For this review, take the finished solid that the model builds, in its own axes (mm). Face numbers are marked on the shaded views. A direction names the side the tool comes from. Coordinates: 2 decimals unless noted, no trailing zeros. Loops run counter-clockwise (first coordinate to the right, second up) from the corner with the lowest first, then second, coordinate; pieces in that order, holes last. Notation, with made-up numbers: M -30,49.5 L 7,49.5 A29 cw 7,70.5 Z; hole C 57,78.25 d7. An arc over 180 degrees is marked long. Answer as a JSON object with one key per item and string values. Group by question number.
Item 1: Mouldability with a two-part tool opening along X and no side actions: class the marked faces 3, 4 and 5 as +X half, -X half, draft (parallel to the pull), parting line (faces both ways), or undercut.
Item 2: Add section B-B (y = -4). State the section outline as (x, z) points, then the cut area to 3 significant figures.
Item 3: Wall thickness on L1, parallel to X at y = -6, z = 22.25; L2, parallel to Y at x = -2, z = 5; L3, parallel to X at y = -2.5, z = 27.25: over which ranges is each line inside the solid? List them lowest first. Write a range as from..to.
Item 4: Add section A-A (z = 10.5). State the section outline as (x, y) points.
Item 5: Add section D-D (z = 6.75). State the section outline as (x, y) points.
Item 6: Add section C-C (y = 0). State the section outline as (x, z) points, then the cut area to 3 significant figures.
Item 7: Tool access review of the marked faces 1 and 2: name each direction out of +Z, -Z, +X, -X, +Y, -Y from which nothing blocks a thin tool from reaching the whole face with its end or side.
Item 8: Insertion check: pin 1 (15 mm diameter, centred on x = -4, z = 17, fed in from -Y); pin 2 (9 mm diameter, centred on x = -13, z = 10.5, fed in from +Y); pin 3 (3.5 mm diameter, centred on x = -22, y = 0.5, fed in from +Z). Each pin has a flat end and moves straight along its axis. Give the tip position at first contact, or say it passes through.
from build123d import *

# Parameters (mm, degrees)
BOSS_EXTRUDE1_DEPTH = 30
SKETCH3_W           = 6
SKETCH3_H           = 3
BOSS_EXTRUDE2_DEPTH = 10
SKETCH4_R           = 3.5
BOSS_EXTRUDE3_DEPTH = 30


with BuildPart() as part:
    # Sketch2 → Boss-Extrude1 (new body)
    with BuildSketch(Plane.XY):
        Polygon((-20, -1.5), (8.5, -1.5), (8.5, -8.5), (10.5, -8.5), (10.5, -1.5), (18, -1.5), (18, -8.5), (20, -8.5), (20, -1.5), (20, 1.5), (-20, 1.5), align=None)
    extrude(amount=BOSS_EXTRUDE1_DEPTH)

    # Sketch3 → Boss-Extrude2 (add)
    with BuildSketch(Plane.XY):
        with Locations((-23, 0)):
            Rectangle(SKETCH3_W, SKETCH3_H)
    extrude(amount=BOSS_EXTRUDE2_DEPTH)

    # Sketch4 → Boss-Extrude3 (add)
    with BuildSketch(Plane.XY):
        with Locations((-27.465142918, 0)):
            Circle(SKETCH4_R)
    extrude(amount=BOSS_EXTRUDE3_DEPTH)


solid = part.part
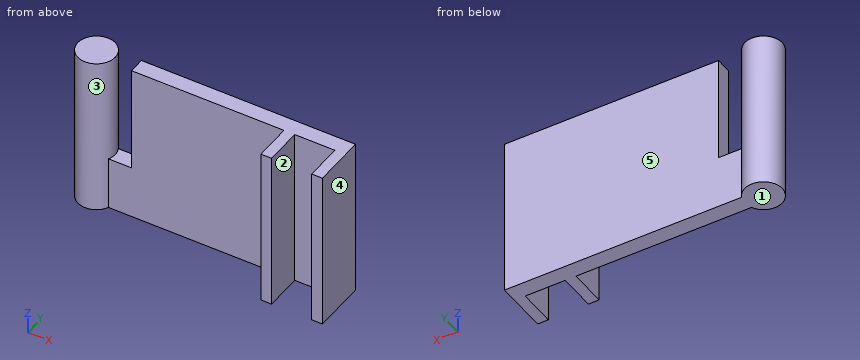
From the geometry:
{
 "1": {"face 3": "undercut", "face 4": "+X half", "face 5": "draft"},
 "2": {"outline": "M 8.5,0 L 10.5,0 L 10.5,30 L 8.5,30 Z; M 18,0 L 20,0 L 20,30 L 18,30 Z", "area": "120 mm²"},
 "3": {"L1": "x = 8.5..10.5, 18..20", "L2": "y = -1.5..1.5", "L3": "x = -29.91..-25.02, 8.5..10.5, 18..20"},
 "4": {"outline": "C -27.47,0 d7; M -20,-1.5 L 8.5,-1.5 L 8.5,-8.5 L 10.5,-8.5 L 10.5,-1.5 L 18,-1.5 L 18,-8.5 L 20,-8.5 L 20,1.5 L -20,1.5 Z"},
 "5": {"outline": "M -24.3,-1.5 L 8.5,-1.5 L 8.5,-8.5 L 10.5,-8.5 L 10.5,-1.5 L 18,-1.5 L 18,-8.5 L 20,-8.5 L 20,1.5 L -24.3,1.5 A3.5 ccw long Z"},
 "6": {"outline": "M -30.97,0 L 20,0 L 20,30 L -20,30 L -20,10 L -23.97,10 L -23.97,30 L -30.97,30 Z", "area": "1,450 mm²"},
 "7": {"face 1": "-Z, +X, -X, +Y, -Y", "face 2": "+Z, -Z, -Y"},
 "8": {"pin 1": "stops at y = -1.5", "pin 2": "stops at y = 1.5", "pin 3": "stops at z = 10"}
}
